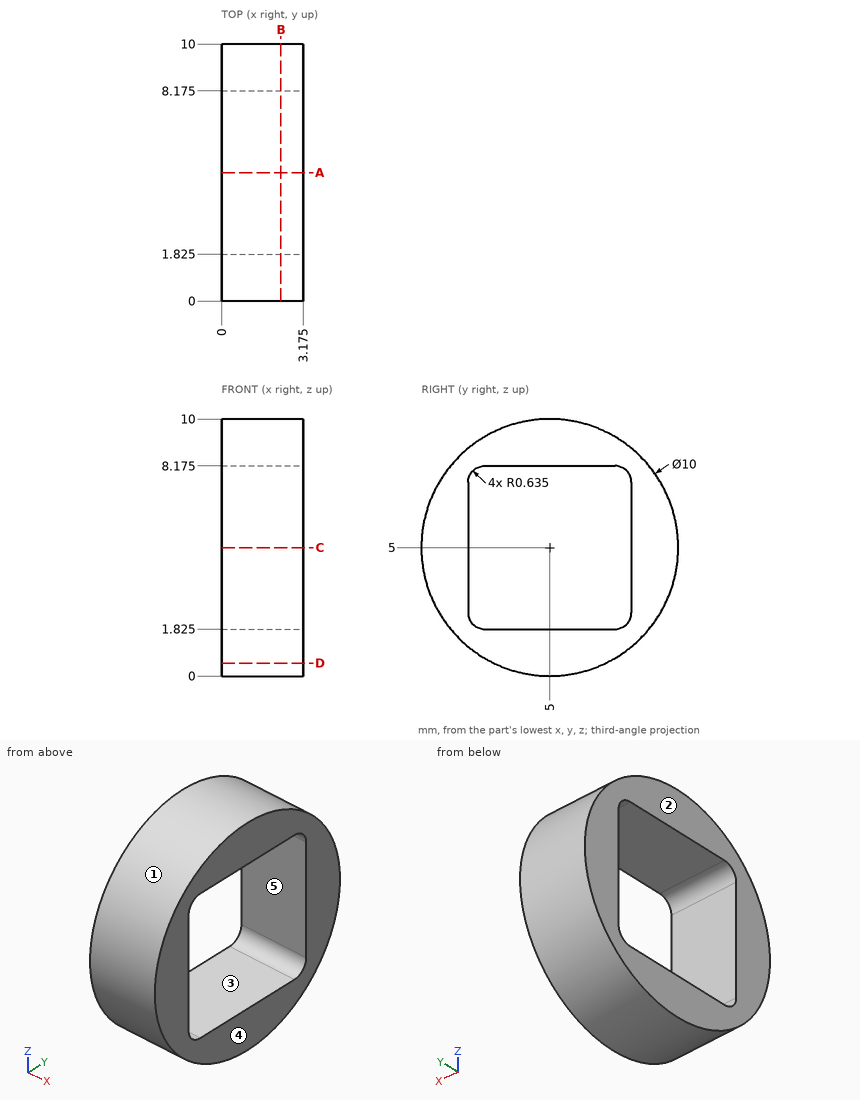
Could you check a few things on this drawing? It's one solid part, dimensions in mm from its lowest x, y, z. A direction names the side the tool comes from. Round coordinates to 2 decimals unless told otherwise and drop trailing zeros. Write each loop counter-clockwise with the first axis right and the second up, starting at its lowest first coordinate (ties: lowest second). Pieces come first, ordered by that corner, then holes.
Q1. Will these pins go through, and if not, where does the flat tip stop? P1, Ø1, axis at x = 1, z = 7.5, coming from the -Y side; P2, Ø1.6, axis at x = 2, z = 4, coming from the -Y side.
Q2. If we section it at D-D on z = 0.5: Write out the boundary of the cut face in (x, y) (3 decimals).
Q3. Please list where these lines run through material, in increasing order: probe 1 along Y at (x, z) = (2, 3) (3 decimals); probe 2 along Y at (x, z) = (2.3, 7.25) (3 decimals); probe 3 along Z at (x, y) = (1.2, 7.5) (3 decimals).
Q4. If we section it at B-B on x = 2.3: Write out the boundary of the cut face in (y, z) (3 decimals).
Q5. Which directions (+Z, -Z, +X, -X, +Y, -Y) give clear straight access to the entire face, cutting with the end or side of a thin tool? Please do the marked faces 4 and 5.
Q6. If we mould it in two halves opening along Y, with no side actions, what happens to the marked faces 1, 2 and 3? For each: +Y half, -Y half, draft (parallel to the pull), parting line (faces both ways), or undercut.
Q7. If we section it at A-A on y = 5: Write out the boundary of the cut face in (x, z) (3 decimals).
Answer below:
1. P1: stops at y = 0.42
1. P2: stops at y = 0
2. outline: (0, 2.821) - (3.175, 2.821) - (3.175, 7.179) - (0, 7.179) - close
3. probe 1: y = 0.417 to 1.825, 8.175 to 9.583
3. probe 2: y = 0.535 to 1.825, 8.175 to 9.465
3. probe 3: z = 0.67 to 1.825, 8.175 to 9.33
4. outline: circle Ø10 at (5, 5); hole (1.825, 2.46) arc R0.635 ccw to (2.46, 1.825) - (7.54, 1.825) arc R0.635 ccw to (8.175, 2.46) - (8.175, 7.54) arc R0.635 ccw to (7.54, 8.175) - (2.46, 8.175) arc R0.635 ccw to (1.825, 7.54) - close
5. face 4: +Z, -Z, +X, +Y, -Y
5. face 5: +X, -X
6. face 1: parting line
6. face 2: draft
6. face 3: undercut
7. outline: (0, 0) - (3.175, 0) - (3.175, 1.825) - (0, 1.825) - close; (0, 8.175) - (3.175, 8.175) - (3.175, 10) - (0, 10) - close
